Build history of the part. All positions in model axes, mm. Face numbers are marked on the shaded views. Coordinates: 2 decimals unless noted, no trailing zeros. Order: outer loops, then holes, each group sorted by start corner. A loop starts at its lowest first (then second) coordinate and runs counter-clockwise, first axis right, second up. Notation, with made-up numbers: (-12.75, 45.5) - (37.25, 45.5) arc R25 cw to (37.25, 68.5) - close; hole circle Ø9 at (62, -16.5). An arc over 180 degrees is marked (long way). Write each question's results on one line, items separated by ' | '. Start each with the question number.
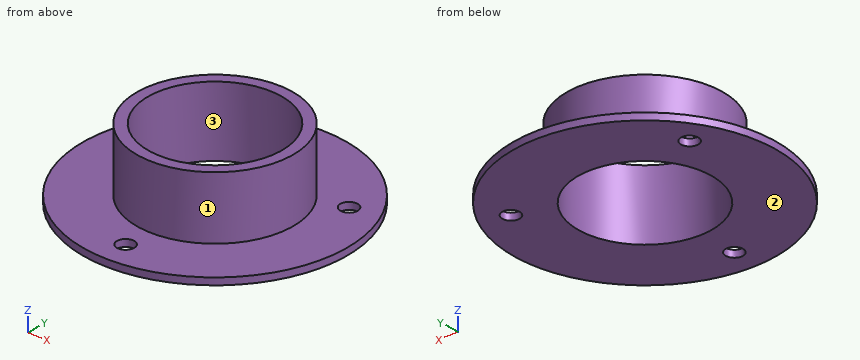
Autodesk Fusion 360 part; units mm, degrees
sketch "Sketch1" plane through (0, 0, 0) normal (0, 0, 1) x (1, 0, 0)
  circle A0 centre (0, 0) radius 19.3
  circle A1 centre (0, 0) radius 22.5
  circle A2 centre (0, 0) radius 38
  dimension "d1" = 45
  dimension "d2" = 38.6
  dimension "d3" = 76
extrude "Extrude1" add sketch "Sketch1" along normal blind 20 contours A1
sketch "Sketch2" plane through (0, 0, 0) normal (0, 0, 1) x (1, 0, 0)
  circle A0 centre (0.2654, -30.1553) radius 2.5
  dimension "d8" = 5
extrude "Extrude4" add sketch "Sketch1" along normal blind 2 contours A1 | A2
extrude "Extrude5" cut sketch "Sketch2" along normal blind 6.312
pattern_circular "C-Pattern2" count 3 over 360 about axis through (0, 0, 2) along (0, 0, 1) of "Extrude5"
Item 1: Slice it at D-D (x = -26.5). Write the cut outline in (y, z), then the cut area to 3 significant figures.
Item 2: Slice it at C-C (z = 17.75). Write the cut outline in (x, y).
Item 3: Slice it at B-B (x = 7.5). Write the cut outline in (y, z), then the cut area to 3 significant figures.
Item 4: Flat gauge pins, fed straight in: P1, Ø10, axis at x = -3, y = -29.5, coming from the +Z side; P2, Ø1.5, axis at x = -2.5, z = 4.5, coming from the +Y side; P3, Ø12, axis at x = -7, z = 7.5, coming from the +Y side; P4, Ø3, axis at x = 25.98, y = 15.31, coming from the -Z side. Where does each tip first touch, or does it go through?
Item 5: Pull direction Y, two halves, no side cores. Call the marked faces 1, 2 and 3: released by +Y, released by -Y, zero draft, split by the parting line, or undercut.
Item 6: Slice it at A-A (y = -3). Write the cut outline in (x, z).
Item 7: Probe probe 1 along X at (y, z) = (-0.5, 12); probe 2 along Z at (x, y) = (25, -24.5); probe 3 along Y at (x, z) = (4.5, 8.5). List the from-to ranges inside material, lowest first.
Resolved:
1) outline: (-27.24, 0) - (12.36, 0) - (12.36, 2) - (-27.24, 2) - close; (17.34, 0) - (27.24, 0) - (27.24, 2) - (17.34, 2) - close | area: 99.0 mm^2
2) outline: circle Ø45 at (0, 0); hole circle Ø38.6 at (0, 0)
3) outline: (-37.25, 0) - (-17.78, 0) - (-17.78, 20) - (-21.21, 20) - (-21.21, 2) - (-37.25, 2) - close; (17.78, 0) - (37.25, 0) - (37.25, 2) - (21.21, 2) - (21.21, 20) - (17.78, 20) - close | area: 201 mm^2
4) P1: z = 2 | P2: y = 22.43 | P3: y = 37.72 | P4: through
5) face 1: split by the parting line | face 2: zero draft | face 3: undercut
6) outline: (-37.88, 0) - (-19.07, 0) - (-19.07, 20) - (-22.3, 20) - (-22.3, 2) - (-37.88, 2) - close; (19.07, 0) - (37.88, 0) - (37.88, 2) - (22.3, 2) - (22.3, 20) - (19.07, 20) - close
7) probe 1: -22.49 to -19.29, 19.29 to 22.49 | probe 2: 0 to 2 | probe 3: -22.05 to -18.77, 18.77 to 22.05
